Autodesk Inventor part; units mm, degrees
ref_plane "YZ Plane" through (0, 0, 0) normal (1, 0, 0) x (0, 1, 0)
ref_plane "XZ Plane" through (0, 0, 0) normal (0, 1, 0) x (-1, 0, 0)
ref_plane "XY Plane" through (0, 0, 0) normal (0, 0, 1) x (1, 0, 0)
sketch "Sketch1" plane through (0, 0, 0) normal (0, 1, 0) x (-1, 0, 0)
  line L0 (-15.875, 15.875) -> (15.875, 15.875)
  line L1 (15.875, 15.875) -> (15.875, -15.875)
  line L2 (15.875, -15.875) -> (-15.875, -15.875)
  line L3 (-15.875, -15.875) -> (-15.875, 15.875)
  line L4 (-15.875, 15.875) -> (15.875, -15.875) construction
  line L5 (15.875, 15.875) -> (-15.875, -15.875) construction
  line L6 (-15.875, 15.875) -> (-12.7, 15.875)
  line L7 (-12.7, 15.875) -> (-12.7, 34.925)
  line L8 (-12.7, 34.925) -> (-15.875, 34.925)
  line L9 (-15.875, 34.925) -> (-15.875, 15.875)
  line L10 (15.875, 15.875) -> (12.7, 15.875)
  line L11 (12.7, 15.875) -> (12.7, 34.925)
  line L12 (12.7, 34.925) -> (15.875, 34.925)
  line L13 (15.875, 34.925) -> (15.875, 15.875)
  point P0 (0, 0)
  dimension "d0" = 31.75
  dimension "d13" = 25.4
  dimension "d14" = 19.05
extrude "Extrusion1" add sketch "Sketch1" along normal mid plane 38.1
sketch "Sketch2" plane through (0, 0, 0) normal (0, 1, 0) x (-1, 0, 0)
  circle A0 centre (0, 0) radius 3.175
  dimension "d3" = 6.35
sketch "Sketch3" plane through (0, 19.05, 0) normal (0, 1, 0) x (1, 0, 0)
  circle A0 centre (0, 0) radius 14.2875
  dimension "d4" = 28.575
sketch "Sketch4" plane through (0, -19.05, 0) normal (0, -1, 0) x (1, 0, 0)
  circle A0 centre (0, 0) radius 14.2875
  dimension "d5" = 28.575
loft "Loft1" cut profiles "Sketch3", "Sketch2", "Sketch4"
fillet "Fillet1" radius 15.875 2 edges at (15.875, 0, -15.875) (-15.875, 0, -15.875)
fillet "Fillet1" radius 12.7 4 edges at (14.2875, 19.05, 34.925) (14.2875, -19.05, 34.925) (-14.2875, 19.05, 34.925) (-14.2875, -19.05, 34.925)
sketch "Sketch5" plane through (-15.875, -19.05, 0) normal (-1, 0, 0) x (0, 0, 1)
  line L0 (15.875, 0) -> (15.875, 38.1) construction
  line L1 (15.875, 0) -> (15.875, 38.1) construction
  circle A0 centre (25.4, 9.525) radius 2.54
  circle A1 centre (25.4, 28.575) radius 2.54
  line L2 (25.4, 9.525) -> (25.4, 28.575) construction
  line L3 (25.4, 19.05) -> (0, 19.05) construction
  dimension "d16" = 5.08
  dimension "d17" = 9.525
  dimension "d18" = 19.05
extrude "Extrusion2" cut sketch "Sketch5" against normal through all
properties part number "climb pull point"
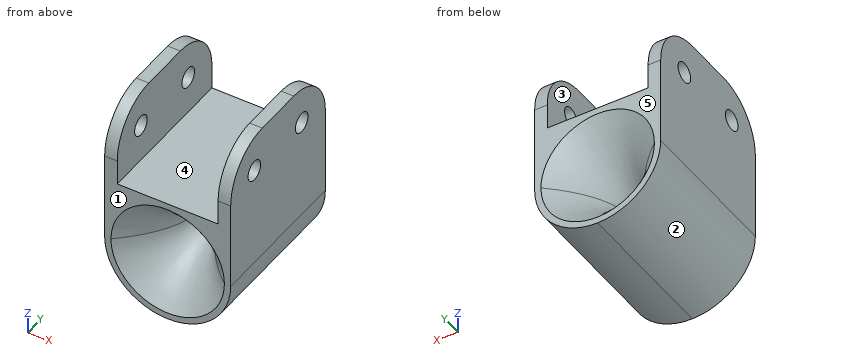
CAD build for the part. Positions are in the model's coordinates, mm. Face numbers are marked on the shaded views. A direction names the side the tool comes from. Round coordinates to 2 decimals unless told otherwise and drop trailing zeros. Order: outer loops, then holes, each group sorted by start corner. A loop starts at its lowest first (then second) coordinate and runs counter-clockwise, first axis right, second up. Notation, with made-up numbers: (-21, 11) - (26, 11) arc R28 ccw to (26, 35) - close; hole circle Ø1 at (9, 24.5). An arc over 180 degrees is marked (long way). Answer as CSV lines item,"result". Start each with the question number.
1. Saw through at B-B, the plane z = 25.4. Write the cut outline in (x, y) (3 decimals).
2. Saw through at A-A, the plane z = 18. Write the cut outline in (x, y) (3 decimals), and give its area (3 significant figures).
3. Tool access for the marked faces 4 and 5: list every direction of +Z, -Z, +X, -X, +Y, -Y with a clear straight run to the whole face (end or side of a thin tool).
4. Pull direction X, two halves, no side cores. Call the marked faces 1, 2 and 3: +X half, -X half, draft (parallel to the pull), parting line (faces both ways), or undercut.
5. Drill centre lines: L1, parallel to X at y = 9.5, z = 29 (3 decimals); L2, parallel to Y at x = 14, z = 25; L3, parallel to Y at x = -15.05, z = 25.4 (3 decimals). Where is each one in solid material? Low to high. Write a range as [from, to].
6. Pin check, flat tips, straight feed: pin 1 (3 mm diameter, centred on y = -6, z = -4.5, fed in from +X); pin 2 (4 mm diameter, centred on y = -4.5, z = -6.5, fed in from +X); pin 3 (4.5 mm diameter, centred on y = 9.525, z = 25.4, fed in from -X); pin 4 (12 mm diameter, centred on x = -12.5, y = -3, fed in from -Z). Stop position of each tip, or through.
7. Saw through at C-C, the plane z = 31. Write the cut outline in (x, y) (3 decimals).
Model answer:
1,outline,"(-15.875, -18.647) - (-12.7, -18.647) - (-12.7, -12.065) - (-15.875, -12.065) - close; (-15.875, -6.985) - (-12.7, -6.985) - (-12.7, 6.985) - (-15.875, 6.985) - close; (-15.875, 12.065) - (-12.7, 12.065) - (-12.7, 18.647) - (-15.875, 18.647) - close; (12.7, -18.647) - (15.875, -18.647) - (15.875, -12.065) - (12.7, -12.065) - close; (12.7, -6.985) - (15.875, -6.985) - (15.875, 6.985) - (12.7, 6.985) - close; (12.7, 12.065) - (15.875, 12.065) - (15.875, 18.647) - (12.7, 18.647) - close"
2,outline,"(-15.875, -19.05) - (-12.7, -19.05) - (-12.7, 19.05) - (-15.875, 19.05) - close; (12.7, -19.05) - (15.875, -19.05) - (15.875, 19.05) - (12.7, 19.05) - close"
2,area,"242 mm²"
3,face 4,"+Z, +Y, -Y"
3,face 5,"+Z, -Z, +X, -X, +Y"
4,face 1,"draft"
4,face 2,"-X half"
4,face 3,"undercut"
5,L1,"x = [-15.875, -12.7], [12.7, 15.875]"
5,L2,"y = [-18.74, -12.03], [-7.02, 7.02], [12.03, 18.74]"
5,L3,"y = [-18.647, -12.065], [-6.985, 6.985], [12.065, 18.647]"
6,pin 1,"stops at x = 15.59"
6,pin 2,"stops at x = 15.22"
6,pin 3,"passes through"
6,pin 4,"stops at z = -14.48"
7,outline,"(-15.875, -15.531) - (-12.7, -15.531) - (-12.7, 15.531) - (-15.875, 15.531) - close; (12.7, -15.531) - (15.875, -15.531) - (15.875, 15.531) - (12.7, 15.531) - close"
